Geometry check sheet. Reference: drawing and pictorial views, mm from the part's lowest x, y, z. Coordinates: 2 decimals unless noted, no trailing zeros. Loops run counter-clockwise (first coordinate to the right, second up) from the corner with the lowest first, then second, coordinate; pieces in that order, holes last. Notation, with made-up numbers: (54.5, -26) - (95.5, -26) arc R17 ccw to (95.5, 6) - close; hole circle Ø2 at (42.25, 61). An arc over 180 degrees is marked (long way). One line per item, written item: value.
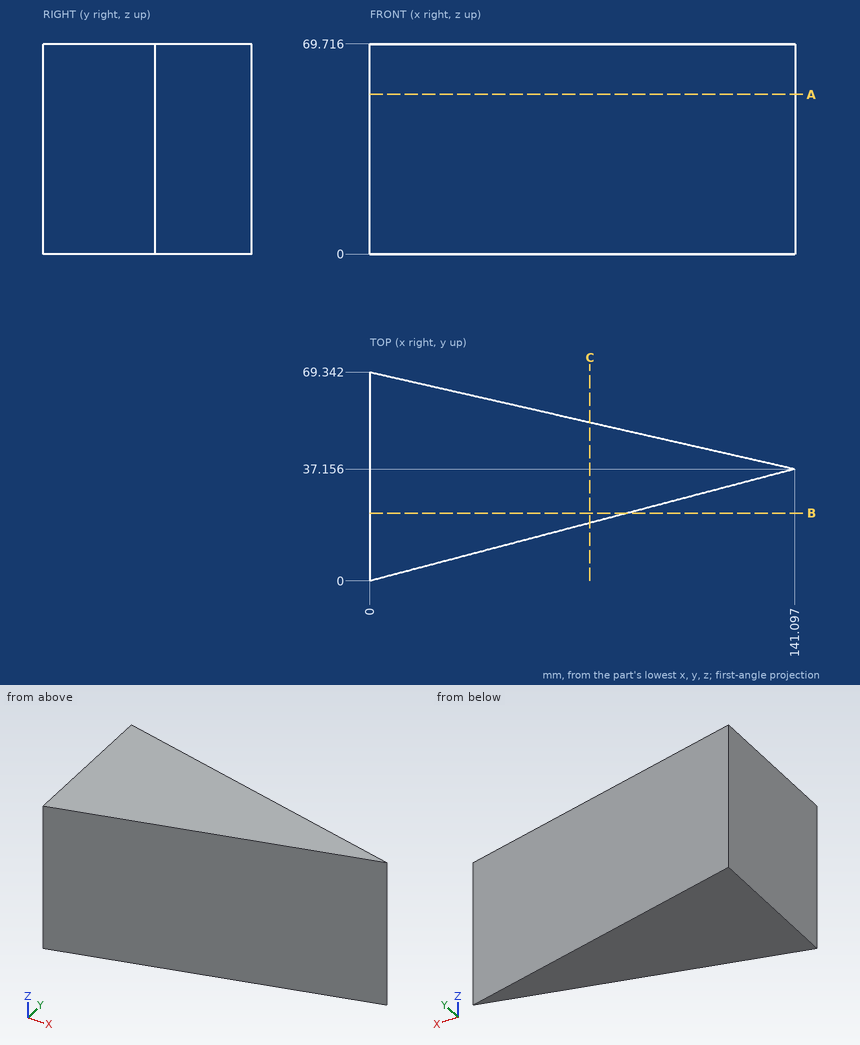
(1) Go/stop test with flat-tipped pins: pin 1 Ø2 at (x, z) = (94.5, 23) entering from -Y; pin 2 Ø1 at (x, z) = (102.5, 57.5) entering from +Y (1 decimal); pin 3 Ø3 at (x, z) = (85, 40) entering from -Y. Record where each tip stops, or that it passes through.
Reply:
pin 1: y = 24.62
pin 2: y = 46.1
pin 3: y = 21.99
(2) Material ranges on probe 1 along Y at (x, z) = (105, 55); probe 2 along Y at (x, z) = (19, 40), recorded low to high. Write a range as from..to.
Reply:
probe 1: 27.65..45.39
probe 2: 5..65.01
(3) Cross-section at A-A on z = 53. Record the cut outline in (x, y) (1 decimal).
Reply:
outline: (0, 0) - (141.1, 37.2) - (0, 69.3) - close
(4) Cross-section at C-C on x = 73. Record the cut outline in (y, z) (1 decimal), and give its area (3 significant figures).
Reply:
outline: (19.2, 0) - (52.7, 0) - (52.7, 69.7) - (19.2, 69.7) - close
area: 2,330 mm2
(5) Cross-section at B-B on y = 22.5. Record the cut outline in (x, z) (1 decimal).
Reply:
outline: (0, 0) - (85.4, 0) - (85.4, 69.7) - (0, 69.7) - close
